Answer from the drawing. Dimensions are ordinates in mm from the lowest x, y and z of the part. A direction names the side the tool comes from. Give positions to 0.01 mm unless a question says otherwise; leave off trailing zeros. Write each loop counter-clockwise with the first axis right and the second up, starting at its lowest first coordinate (ties: lowest second). Pieces come first, ordered by that corner, then holes. Notation, with made-up numbers: (56, -38.5) -> (94, -38.5) arc R27 ccw to (94, -15.5) -> close; hole circle Ø2 at (26, 63.25). An arc over 180 degrees is marked (long way). Put each result on its own line as item: value. Start each with the question number.
1) A cutting plane is placed at D-D (x = 25). Write down the section's boundary in (y, z), then the cut area to 3 significant figures.
2) For a pull along Y with two mould halves and no side action, classify the marked faces 6, 7 and 8 as released by +Y, released by -Y, zero draft, split by the parting line, or undercut.
3) Find the intervals of material crossed by line 1 along Z through (x, y) = (43, 11.5); line 2 along Z through (x, y) = (43, 31); line 3 along Y through (x, z) = (31.5, 32) (1 decimal), in increasing order. Write a range as from..to.
4) Flat-ended cylindrical pins translate along their axes: pin 1 Ø6.5 at (x, z) = (6.5, 20) entering from -Y; pin 2 Ø3 at (x, z) = (43, 39) entering from -Y; pin 3 Ø14 at (x, y) = (26.5, 24.5) entering from -Z; pin 4 Ø12 at (y, z) = (28, 26) entering from -X. Find the tip coordinate at first contact, or state that the pin passes through.
5) For the marked faces 1, 2, 3, 4 and 5, determine the directions among +Z, -Z, +X, -X, +Y, -Y from which every point of the face is accessible in a straight line to the end or side of a thin tool.
6) A cutting plane is placed at A-A (y = 19.5). Write down the section's boundary in (x, z), then the cut area to 3 significant figures.
7) A cutting plane is placed at C-C (z = 39). Give the number of separate pieces and of enclosed holes in the cut face, then the cut area to 3 significant figures.
8) A cutting plane is placed at B-B (x = 7). Write down the section's boundary in (y, z).
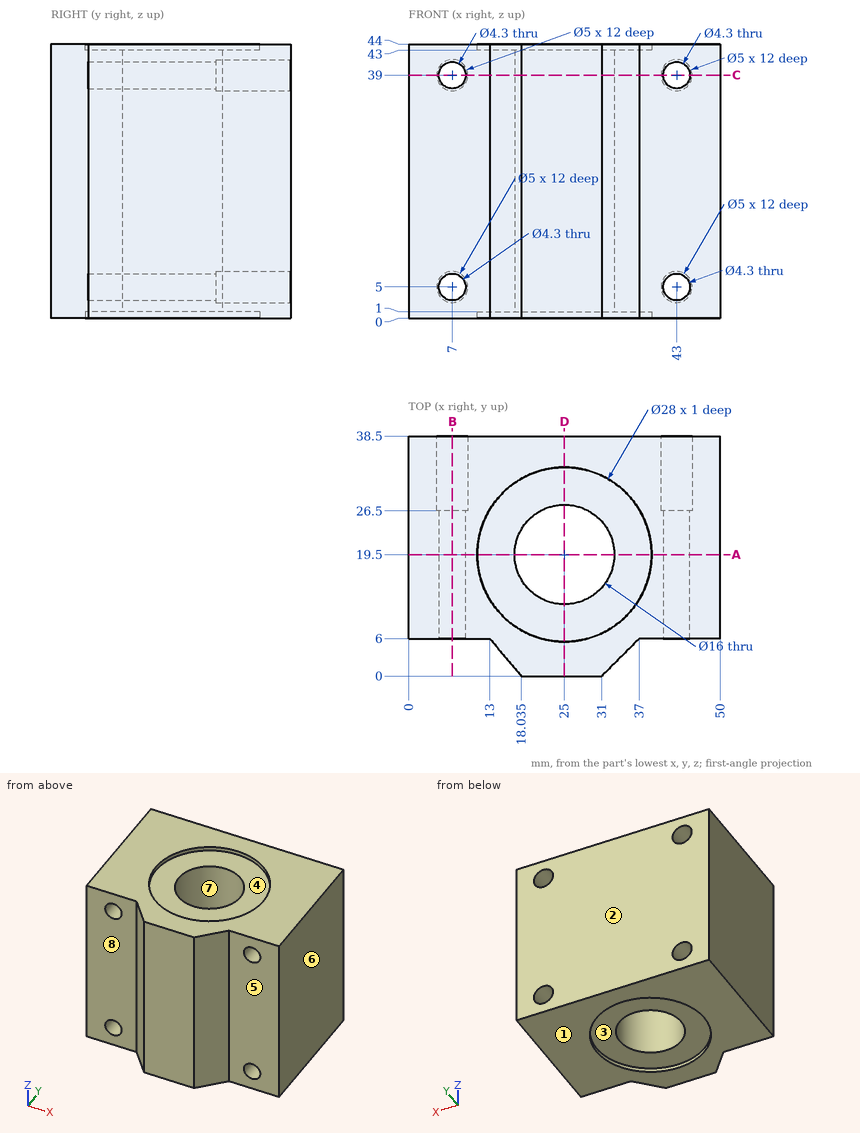
Reply:
1. outline: (0, 0) -> (5.5, 0) -> (5.5, 1) -> (11.5, 1) -> (11.5, 43) -> (5.5, 43) -> (5.5, 44) -> (0, 44) -> close; (27.5, 1) -> (33.5, 1) -> (33.5, 0) -> (38.5, 0) -> (38.5, 44) -> (33.5, 44) -> (33.5, 43) -> (27.5, 43) -> close
1. area: 966 mm2
2. face 6: zero draft
2. face 7: undercut
2. face 8: released by -Y
3. line 1: z = 0..2.85, 7.15..36.85, 41.15..44
3. line 2: z = 0..2.5, 7.5..36.5, 41.5..44
3. line 3: y = 0.5..14.8, 24.2..38.5
4. pin 1: stops at y = 6
4. pin 2: passes through
4. pin 3: stops at z = 1
4. pin 4: stops at x = 0
5. face 1: -Z, +X, -X, +Y, -Y
5. face 2: +Z, -Z, +X, -X, +Y
5. face 3: -Z
5. face 4: +Z
5. face 5: +Z, -Z, +X, -Y
6. outline: (0, 0) -> (11, 0) -> (11, 1) -> (17, 1) -> (17, 43) -> (11, 43) -> (11, 44) -> (0, 44) -> close; (33, 1) -> (39, 1) -> (39, 0) -> (50, 0) -> (50, 44) -> (39, 44) -> (39, 43) -> (33, 43) -> close; hole circle Ø4.3 at (7, 5); hole circle Ø4.3 at (7, 39); hole circle Ø4.3 at (43, 5); hole circle Ø4.3 at (43, 39)
6. area: 1,410 mm2
7. separate pieces: 3
7. enclosed holes: 1
7. area: 1,240 mm2
8. outline: (6, 0) -> (38.5, 0) -> (38.5, 2.5) -> (26.5, 2.5) -> (26.5, 2.85) -> (6, 2.85) -> close; (6, 7.15) -> (26.5, 7.15) -> (26.5, 7.5) -> (38.5, 7.5) -> (38.5, 36.5) -> (26.5, 36.5) -> (26.5, 36.85) -> (6, 36.85) -> close; (6, 41.15) -> (26.5, 41.15) -> (26.5, 41.5) -> (38.5, 41.5) -> (38.5, 44) -> (6, 44) -> close
